The model under review builds one solid part; all positions refer to its coordinate system, in mm. A direction names the side the tool comes from. Round coordinates to 2 decimals unless told otherwise and drop trailing zeros. Order: outer loops, then holes, each group sorted by start corner. A loop starts at its lowest first (then second) coordinate and runs counter-clockwise, first axis right, second up.
1) To check wall thickness, follow L1, parallel to X at y = 31.2, z = 0; L2, parallel to Y at x = 1, z = 33; L3, parallel to Y at x = -64, z = 28.5. State the ranges of each line that lie inside material, in increasing order.
2) Consider section C-C (y = 46). Give the boundary of the cut face in (x, z).
3) Machinability: for faces 4 (the face through (1, 52, 0)), 5 (the face through (-3, 44, 0)), 6 (the face through (0, 30, -44)), 7 (the face through (-58, 30, -1)), which of the approach directions +Z, -Z, +X, -X, +Y, -Y give a long, thin tool a straight path to every point of the face, cutting with its end or side? Answer none if there is none.
4) Consider section A-A (z = 0). Give the number of separate pieces and of enclosed holes in the cut face, then the cut area to 3 significant figures.
5) Consider section B-B (x = -40.5). Give the boundary of the cut face in (y, z).
6) Clearance check with flat-ended pins moving along their axes: P1, Ø10, axis at y = 21, z = 15, coming from the +X side; P2, Ø5, axis at x = 13.5, z = 47, coming from the +Y side; P3, Ø22.5, axis at x = 48, z = -3.5, coming from the -Y side; P4, Ø2, axis at x = -18, z = 13.5, coming from the +Y side. State where each tip first meets the part, or that it passes through.
7) Consider section D-D (x = 18). Give the boundary of the cut face in (y, z).
8) Mouldability with a two-part tool opening along Z and no side actions: class faces 1 (the face through (-1, 62, 0)), 2 (the face through (-66.905, 30.76, -0.867)), 3 (the face through (-65.979, 30.993, -31.445)) as pulls with the +Z half, pulls with the -Z half, needs draft (parallel to the pull), parting line crosses it, or undercut.
from build123d import *

# Parameters (mm, degrees)
ESBO_O1_R                = 50
RESSALTO_EXTRUS_O1_DEPTH = 30
RESSALTO_EXTRUS_O2_DEPTH = 2
ESBO_O3_R                = 3
RESSALTO_EXTRUS_O3_DEPTH = 30
ESBO_O4_W                = 2.913486889
ESBO_O4_H                = 6.765215319
CORTE_EXTRUS_O1_DEPTH    = 20
CORTE_EXTRUS_O2_REACH    = 97.65
ESBO_O6_R                = 4
FILETE2_R                = 0.5


with BuildPart() as part:
    # Esboço1 → Ressalto-extrusão1 (new body)
    with BuildSketch(Plane(origin=(0, 0, 0), x_dir=(1, 0, 0), z_dir=(0, 1, 0))):
        with Locations(Location((0, 0, 0), (0, 0, 270))):
            Circle(ESBO_O1_R)
    extrude(amount=RESSALTO_EXTRUS_O1_DEPTH)

    # Esboço2 → Ressalto-extrusão2 (add)
    with BuildSketch(Plane(origin=(0, 30, 0), x_dir=(1, 0, 0), z_dir=(0, 1, 0))):
        with BuildLine():
            Line((-45, -40), (45, -40))
            ThreePointArc((45, -40), (66.213203436, -31.213203436), (75, -10))
            Line((75, -10), (75, 10))
            ThreePointArc((75, 10), (66.213203436, 31.213203436), (45, 40))
            Line((45, 40), (-45, 40))
            ThreePointArc((-45, 40), (-66.213203436, 31.213203436), (-75, 10))
            Line((-75, 10), (-75, -10))
            ThreePointArc((-75, -10), (-66.213203436, -31.213203436), (-45, -40))
        make_face()
    extrude(amount=RESSALTO_EXTRUS_O2_DEPTH)

    # Esboço3 → Ressalto-extrusão3 (add)
    with BuildSketch(Plane(origin=(0, 32, 0), x_dir=(1, 0, 0), z_dir=(0, 1, 0))):
        with Locations(Location((0, 0, 0), (0, 0, 90))):
            Circle(ESBO_O3_R)
    extrude(amount=RESSALTO_EXTRUS_O3_DEPTH)

    # Esboço4 → Corte-extrusão1 (cut)
    with BuildSketch(Plane(origin=(0, 62, 0), x_dir=(1, 0, 0), z_dir=(0, 1, 0))):
        with Locations((2.456743444, -0.010763652)):
            Rectangle(ESBO_O4_W, ESBO_O4_H)
    extrude(amount=-CORTE_EXTRUS_O1_DEPTH, mode=Mode.SUBTRACT)

    # Esboço6 → Corte-extrusão2 (cut, up to next)
    with BuildSketch(Plane(origin=(0, 32, 0), x_dir=(1, 0, 0), z_dir=(0, 1, 0)), mode=Mode.PRIVATE) as corte_extrus_o2_sk1:
        with Locations(Location((-63, 0, 0), (0, 0, 270))):
            Circle(ESBO_O6_R)
    corte_extrus_o2_tool1 = extrude(corte_extrus_o2_sk1.sketch, amount=-CORTE_EXTRUS_O2_REACH, mode=Mode.PRIVATE) & part.part
    # Esboço6 → Corte-extrusão2 (cut, up to next)
    with BuildSketch(Plane(origin=(0, 32, 0), x_dir=(1, 0, 0), z_dir=(0, 1, 0)), mode=Mode.PRIVATE) as corte_extrus_o2_sk2:
        with Locations(Location((63, 0, 0), (0, 0, 90))):
            Circle(ESBO_O6_R)
    corte_extrus_o2_tool2 = extrude(corte_extrus_o2_sk2.sketch, amount=-CORTE_EXTRUS_O2_REACH, mode=Mode.PRIVATE) & part.part
    add(corte_extrus_o2_tool1.solids().sort_by_distance((-63, 32, 0))[0], mode=Mode.SUBTRACT)
    add(corte_extrus_o2_tool2.solids().sort_by_distance((63, 32, 0))[0], mode=Mode.SUBTRACT)

    # Filete2
    # the kernel refuses this fillet: 0.5 mm, written as the material it adds along each edge
    with BuildSketch(Plane(origin=(0, 32, 0), x_dir=(0, 0, -1), z_dir=(1, 0, 0))) as filete2_piece_1:
        with BuildLine():
            CenterArc((3 + FILETE2_R, FILETE2_R), FILETE2_R, 180, 90)
            Line((3, FILETE2_R), (3, 0))
            Line((3, 0), (3 + FILETE2_R, 0))
        make_face()
    revolve(axis=Axis((0, 32, 0), (0, 1, 0)))
    # the kernel refuses this fillet: 0.5 mm, written as the material it takes off along each edge
    with BuildSketch(Plane(origin=(-45, 30, 40), x_dir=(0, 0, -1), z_dir=(1, 0, 0))) as filete2_2_piece_1_section:
        with BuildLine():
            CenterArc((FILETE2_R, FILETE2_R), FILETE2_R, 180, 90)
            Line((0, FILETE2_R), (0, 0))
            Line((0, 0), (FILETE2_R, 0))
        make_face()
    filete2_2_piece_1 = extrude(amount=16.25, mode=Mode.PRIVATE)
    filete2_2_piece_1 = filete2_2_piece_1 - Plane(origin=(0, 30.083724815, 0), x_dir=(0, 0, 1), z_dir=(0, -1, 0)) * Cylinder(50, 35, mode=Mode.PRIVATE)
    add(filete2_2_piece_1, mode=Mode.SUBTRACT)
    with BuildSketch(Plane(origin=(45, 32, -10), x_dir=(1, 0, 0), z_dir=(0, 0, 1))) as filete2_2_piece_2:
        with BuildLine():
            CenterArc((30 - FILETE2_R, -FILETE2_R), FILETE2_R, 0, 90)
            Line((30 - FILETE2_R, 0), (30, 0))
            Line((30, 0), (30, -FILETE2_R))
        make_face()
    revolve(axis=Axis((45, 32, -10), (0, 1, 0)), revolution_arc=90, mode=Mode.SUBTRACT)
    with BuildSketch(Plane(origin=(45, 32, -40), x_dir=(0, -1, 0), z_dir=(-1, 0, 0)), Plane(origin=(-45, 32, 40), x_dir=(0, -1, 0), z_dir=(1, 0, 0))) as filete2_2_piece_3:
        with BuildLine():
            CenterArc((FILETE2_R, FILETE2_R), FILETE2_R, 180, 90)
            Line((0, FILETE2_R), (0, 0))
            Line((0, 0), (FILETE2_R, 0))
        make_face()
    extrude(amount=90, mode=Mode.SUBTRACT)
    with BuildSketch(Plane(origin=(-45, 32, -10), x_dir=(0, 0, -1), z_dir=(1, 0, 0))) as filete2_2_piece_4:
        with BuildLine():
            CenterArc((30 - FILETE2_R, -FILETE2_R), FILETE2_R, 0, 90)
            Line((30 - FILETE2_R, 0), (30, 0))
            Line((30, 0), (30, -FILETE2_R))
        make_face()
    revolve(axis=Axis((-45, 32, -10), (0, 1, 0)), revolution_arc=90, mode=Mode.SUBTRACT)
    with BuildSketch(Plane(origin=(-75, 32, -10), x_dir=(0, -1, 0), z_dir=(0, 0, 1)), Plane(origin=(75, 32, 10), x_dir=(0, -1, 0), z_dir=(0, 0, -1)), Plane(origin=(-75, 30, -10), x_dir=(1, 0, 0), z_dir=(0, 0, 1))) as filete2_2_piece_5:
        with BuildLine():
            CenterArc((FILETE2_R, FILETE2_R), FILETE2_R, 180, 90)
            Line((0, FILETE2_R), (0, 0))
            Line((0, 0), (FILETE2_R, 0))
        make_face()
    extrude(amount=20, mode=Mode.SUBTRACT)
    with BuildSketch(Plane(origin=(-45, 32, 10), x_dir=(-1, 0, 0), z_dir=(0, 0, -1))) as filete2_2_piece_6:
        with BuildLine():
            CenterArc((30 - FILETE2_R, -FILETE2_R), FILETE2_R, 0, 90)
            Line((30 - FILETE2_R, 0), (30, 0))
            Line((30, 0), (30, -FILETE2_R))
        make_face()
    revolve(axis=Axis((-45, 32, 10), (0, 1, 0)), revolution_arc=90, mode=Mode.SUBTRACT)
    with BuildSketch(Plane(origin=(45, 32, 10), x_dir=(0, 0, 1), z_dir=(-1, 0, 0))) as filete2_2_piece_7:
        with BuildLine():
            CenterArc((30 - FILETE2_R, -FILETE2_R), FILETE2_R, 0, 90)
            Line((30 - FILETE2_R, 0), (30, 0))
            Line((30, 0), (30, -FILETE2_R))
        make_face()
    revolve(axis=Axis((45, 32, 10), (0, 1, 0)), revolution_arc=90, mode=Mode.SUBTRACT)
    with BuildSketch(Plane(origin=(-63, 32, 0), x_dir=(0, 0, 1), z_dir=(-1, 0, 0))) as filete2_2_piece_8:
        with BuildLine():
            CenterArc((4 + FILETE2_R, -FILETE2_R), FILETE2_R, 90, 90)
            Line((4 + FILETE2_R, 0), (4, 0))
            Line((4, 0), (4, -FILETE2_R))
        make_face()
    revolve(axis=Axis((-63, 32, 0), (0, 1, 0)), mode=Mode.SUBTRACT)
    with BuildSketch(Plane(origin=(63, 32, 0), x_dir=(0, 0, -1), z_dir=(1, 0, 0))) as filete2_2_piece_9:
        with BuildLine():
            CenterArc((4 + FILETE2_R, -FILETE2_R), FILETE2_R, 90, 90)
            Line((4 + FILETE2_R, 0), (4, 0))
            Line((4, 0), (4, -FILETE2_R))
        make_face()
    revolve(axis=Axis((63, 32, 0), (0, 1, 0)), mode=Mode.SUBTRACT)
    with BuildSketch(Plane(origin=(-28.75, 30, -40), x_dir=(0, 0, 1), z_dir=(-1, 0, 0))) as filete2_2_piece_10_section:
        with BuildLine():
            CenterArc((FILETE2_R, FILETE2_R), FILETE2_R, 180, 90)
            Line((0, FILETE2_R), (0, 0))
            Line((0, 0), (FILETE2_R, 0))
        make_face()
    filete2_2_piece_10 = extrude(amount=16.25, mode=Mode.PRIVATE)
    filete2_2_piece_10 = filete2_2_piece_10 - Plane(origin=(0, 30.117437767, 0), x_dir=(0, 0, 1), z_dir=(0, -1, 0)) * Cylinder(50, 35, mode=Mode.PRIVATE)
    add(filete2_2_piece_10, mode=Mode.SUBTRACT)
    with BuildSketch(Plane(origin=(-45, 30, -10), x_dir=(0, 0, -1), z_dir=(1, 0, 0))) as filete2_2_piece_11:
        with BuildLine():
            CenterArc((30 - FILETE2_R, FILETE2_R), FILETE2_R, 270, 90)
            Line((30, FILETE2_R), (30, 0))
            Line((30, 0), (30 - FILETE2_R, 0))
        make_face()
    revolve(axis=Axis((-45, 30, -10), (0, 1, 0)), revolution_arc=90, mode=Mode.SUBTRACT)
    with BuildSketch(Plane(origin=(-45, 30, 10), x_dir=(-1, 0, 0), z_dir=(0, 0, -1))) as filete2_2_piece_12:
        with BuildLine():
            CenterArc((30 - FILETE2_R, FILETE2_R), FILETE2_R, 270, 90)
            Line((30, FILETE2_R), (30, 0))
            Line((30, 0), (30 - FILETE2_R, 0))
        make_face()
    revolve(axis=Axis((-45, 30, 10), (0, 1, 0)), revolution_arc=90, mode=Mode.SUBTRACT)


solid = part.part
Answer below:
1. L1: x = -75 to -67, -59 to 59, 67 to 75
1. L2: y = 0 to 32
1. L3: y = 30 to 32
2. outline: (1, -2.83) - (1, 2.83) arc R3 ccw (long way) to start
3. face 4: +Z, -Z, +X, +Y
3. face 5: +Y
3. face 6: -Z, +X, -X, +Y
3. face 7: -X, -Y
4. separate pieces: 3
4. enclosed holes: 0
4. area: 3,410 mm2
5. outline: (0, -29.32) - (30, -29.32) - (30, -39.5) arc R0.5 ccw to (30.5, -40) - (31.5, -40) arc R0.5 ccw to (32, -39.5) - (32, 39.5) arc R0.5 ccw to (31.5, 40) - (30.5, 40) arc R0.5 ccw to (30, 39.5) - (30, 29.32) - (0, 29.32) - close
6. P1: stops at x = 48.99
6. P2: stops at y = 30
6. P3: stops at y = 0
6. P4: stops at y = 32
7. outline: (0, -46.65) - (30, -46.65) - (30, -40) - (31.5, -40) arc R0.5 ccw to (32, -39.5) - (32, 39.5) arc R0.5 ccw to (31.5, 40) - (30, 40) - (30, 46.65) - (0, 46.65) - close
8. face 1: needs draft
8. face 2: undercut
8. face 3: pulls with the -Z half
